Here's how the part is built. I have some questions about the finished solid (model axes, mm). Face numbers are marked on the shaded views. A direction names the side the tool comes from. Round coordinates to 2 decimals unless told otherwise and drop trailing zeros. Loops run counter-clockwise (first coordinate to the right, second up) from the corner with the lowest first, then second, coordinate; pieces in that order, holes last. Notation, with made-up numbers: (21.25, 48.5) - (55.25, 48.5) arc R31 cw to (55.25, 83.5) - close; hole circle Ø10 at (28, -27.75). An arc over 180 degrees is marked (long way). Answer as a JSON object with one key per item and string values. Group by question number.
1) I want a section at A-A, the plane x = 12.75. Please give me the cut outline in (y, z).
2) I want a section at B-B, the plane y = 9. Please give me the cut outline in (x, z).
3) If I drill on line 1 along Z through (x, y) = (2.75, 5.75); line 2 along Y through (x, z) = (16.75, 6.75); line 3 along Y through (x, z) = (9, 0.75), over which ranges is the centre line in solid material (lowest first)? Write a range as [from, to].
4) I want a section at C-C, the plane z = 3.5. Please give me the cut outline in (x, y), then the cut area to 3 significant figures.
5) Will these pins go through, and if not, where does the flat tip stop? P1, Ø1.5, axis at x = 2, y = 11, coming from the -Z side; P2, Ø4, axis at x = 11, z = 5.5, coming from the -Y side; P3, Ø5, axis at x = 6.5, y = 3, coming from the +Z side.
6) Which directions (+Z, -Z, +X, -X, +Y, -Y) give clear straight access to the entire face, cutting with the end or side of a thin tool? Please do the marked faces 1 and 2.
from build123d import *

# Parameters (mm, degrees)
SKETCH_1_W            = 20
SKETCH_1_H            = 10
BASEPLATE_DEPTH       = 1
EDGEFLANGE_DEPTH      = 20
EDGEFLANGE_START      = 1
EDGEFLANGE_FLAT_DEPTH = 1


# Sheet-metal steps are written as plain solids
with BuildPart() as part:
    # Sketch 1 → BasePlate (new body)
    with BuildSketch(Plane.XY):
        with Locations((10, 5)):
            Rectangle(SKETCH_1_W, SKETCH_1_H)
    extrude(amount=-BASEPLATE_DEPTH)

    # EdgeFlange bend section (across the edge) → EdgeFlange (add)
    with BuildSketch(Plane(origin=(20, 12, 0), x_dir=(0, -1, 0), z_dir=(-1, 0, 0))):
        with BuildLine():
            Line((-1, 2), (0, 2))
            ThreePointArc((0, 2), (0.585786438, 0.585786438), (2, 0))
            Line((2, 0), (2, -1))
            ThreePointArc((2, -1), (-0.121320344, -0.121320344), (-1, 2))
        make_face()
    extrude(amount=EDGEFLANGE_DEPTH)

    # EdgeFlange profile (on flange) → EdgeFlange flat (add)
    with BuildSketch(Plane(origin=(0, 12, 0), x_dir=(-1, 0, 0), z_dir=(0, 1, 0)).offset(EDGEFLANGE_START)):
        Polygon((-20, 10), (-20, 2), (0, 2), (0, 10), (-2, 10), (-18, 10), align=None)
    extrude(amount=-EDGEFLANGE_FLAT_DEPTH)


solid = part.part
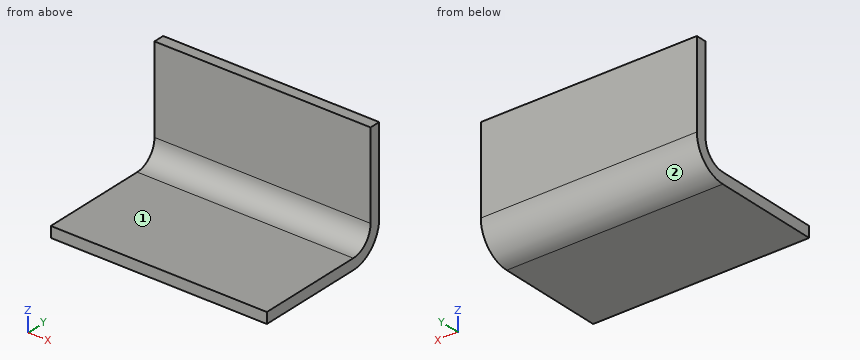
Outcome:
{
 "1": {"outline": "(0, -1) - (10, -1) arc R3 ccw to (13, 2) - (13, 10) - (12, 10) - (12, 2) arc R2 cw to (10, 0) - (0, 0) - close"},
 "2": {"outline": "(0, -1) - (20, -1) - (20, 0) - (0, 0) - close"},
 "3": {"line 1": "[-1, 0]", "line 2": "[12, 13]", "line 3": "[11.56, 12.73]"},
 "4": {"outline": "(0, 12) - (20, 12) - (20, 13) - (0, 13) - close", "area": "20.0 mm^2"},
 "5": {"P1": "z = -0.99", "P2": "y = 12", "P3": "z = 0"},
 "6": {"face 1": "+Z, +X, -X, -Y", "face 2": "-Z, +X, -X, +Y"}
}
